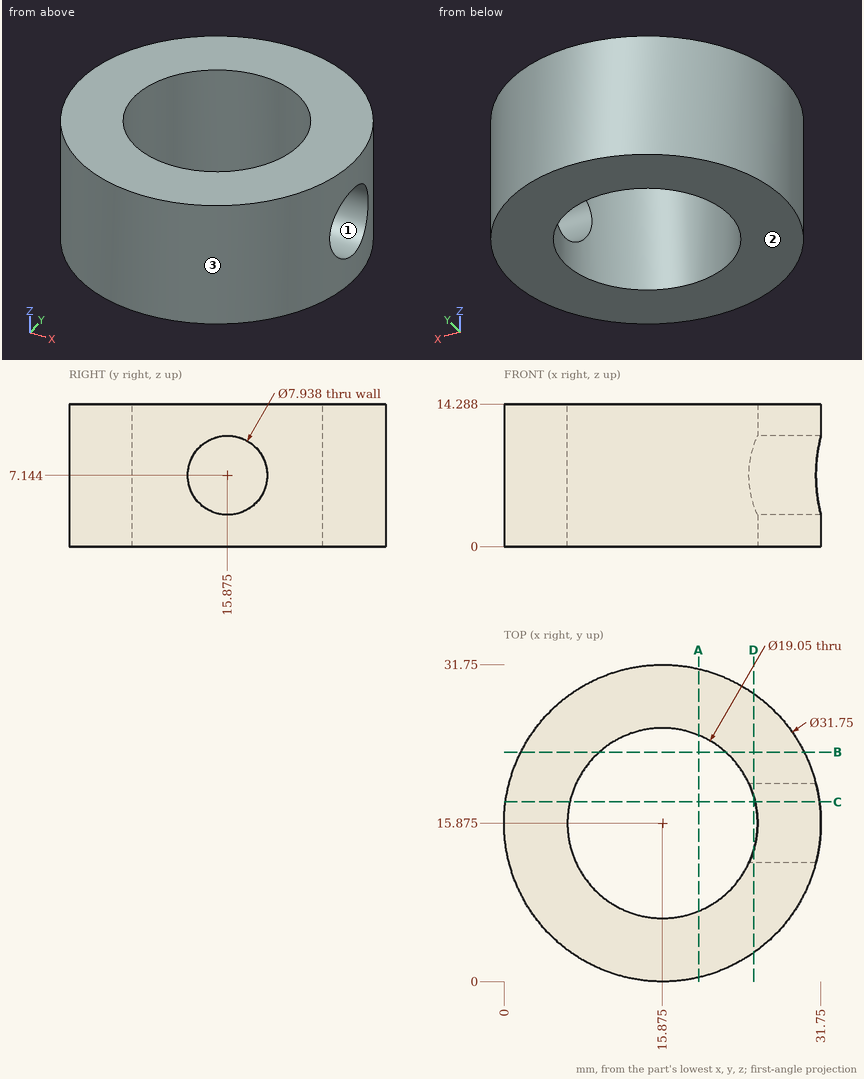
Could you check a few things on this drawing? It's one solid part, dimensions in mm from its lowest x, y, z. Coordinates: 2 decimals unless noted, no trailing zeros. Order: outer loops, then holes, each group sorted by start corner. A loop starts at its lowest first (then second) coordinate and runs counter-clockwise, first axis right, second up. Notation, with made-up numbers: (83.5, 8.25) -> (116.5, 8.25) arc R19 ccw to (116.5, 18.25) -> close; hole circle Ø5 at (21, 35). An arc over 180 degrees is marked (long way). One line per item, written item: value. Start each with the question number.
1) I'm going to push flat-ended pins straight in: pin 1 (3 mm diameter, centred on y = 25.5, z = 2.5, fed in from +X); pin 2 (4 mm diameter, centred on x = 17, y = 23, fed in from -Z); pin 3 (6 mm diameter, centred on y = 5.5, z = 7.5, fed in from -X). Where does each tip first touch, or does it pass through?
2) Imagine slicing it at C-C on y = 18. List the corners of the cut face in (x, z) for me (1 decimal).
3) We'd pull the mould along Y, two halves only. Please class the marked faces 1, 2 and 3: +Y half, -Y half, draft (parallel to the pull), parting line (faces both ways), or undercut.
4) Imagine slicing it at D-D on x = 25. List the corners of the cut face in (y, z) for me (1 decimal).
5) Imagine slicing it at B-B on y = 23. List the corners of the cut face in (x, z) for me.
6) If I drill on L1, parallel to Y at x = 19, z = 11.25; L2, parallel to X at y = 17.5, z = 13.5; L3, parallel to Y at x = 14, z = 4.25 (1 decimal), over which ranges is the centre line in solid material (lowest first)? Write a range as [from, to].
7) Imagine slicing it at A-A on x = 19.5. List the corners of the cut face in (y, z) for me, plus the area to 3 significant figures.
Answer list:
1. pin 1: stops at x = 29.51
1. pin 2: passes through
1. pin 3: stops at x = 1.82
2. outline: (0.1, 0) -> (6.6, 0) -> (6.6, 14.3) -> (0.1, 14.3) -> close; (25.2, 0) -> (31.6, 0) -> (31.6, 3.8) -> (25.2, 3.8) -> close; (25.2, 10.5) -> (31.6, 10.5) -> (31.6, 14.3) -> (25.2, 14.3) -> close
3. face 1: undercut
3. face 2: draft
3. face 3: parting line
4. outline: (2.9, 0) -> (13.1, 0) -> (13.1, 4.3) arc R4 cw to (13.1, 10) -> (13.1, 14.3) -> (2.9, 14.3) -> close; (18.6, 0) -> (28.9, 0) -> (28.9, 14.3) -> (18.6, 14.3) -> (18.6, 10) arc R4 cw to (18.6, 4.3) -> close
5. outline: (1.69, 0) -> (9.55, 0) -> (9.55, 14.29) -> (1.69, 14.29) -> close; (22.2, 0) -> (30.06, 0) -> (30.06, 14.29) -> (22.2, 14.29) -> close
6. L1: y = [0.31, 6.88], [24.87, 31.44]
6. L2: x = [0.08, 6.49], [25.26, 31.67]
6. L3: y = [0.1, 6.5], [25.2, 31.6]
7. outline: (0.42, 0) -> (7.07, 0) -> (7.07, 14.29) -> (0.42, 14.29) -> close; (24.68, 0) -> (31.33, 0) -> (31.33, 14.29) -> (24.68, 14.29) -> close
7. area: 190 mm2
